from build123d import *

# Parameters (mm, degrees)
IZIM1_R                     = 3
Y_KSEKLIK_EKSTR_ZYON1_DEPTH = 3
IZIM2_R                     = 1.5
Y_KSEKLIK_EKSTR_ZYON2_DEPTH = 5
RADYUS1_R                   = 0.5
KES_EKSTR_ZYON1_DEPTH       = 2


with BuildPart() as part:
    # Çizim1 → Yükseklik-Ekstrüzyon1 (new body)
    with BuildSketch(Plane(origin=(0, 0, 0), x_dir=(1, 0, 0), z_dir=(0, 1, 0))):
        with Locations(Location((0, 0, 0), (0, 0, 270))):
            Circle(IZIM1_R)
    extrude(amount=Y_KSEKLIK_EKSTR_ZYON1_DEPTH)

    # Çizim2 → Yükseklik-Ekstrüzyon2 (add)
    with BuildSketch(Plane(origin=(0, 3, 0), x_dir=(1, 0, 0), z_dir=(0, 1, 0))):
        with Locations(Location((0, 0, 0), (0, 0, 270))):
            Circle(IZIM2_R)
    extrude(amount=Y_KSEKLIK_EKSTR_ZYON2_DEPTH)

    # Radyus1
    radyus1_edges = [part.edges().sort_by_distance(p)[0] for p in [
        (0, 0, -3),
        (0, 3, -3),
    ]]
    fillet(radyus1_edges, radius=RADYUS1_R)

    # Çizim3 → Kes-Ekstrüzyon1 (cut)
    with BuildSketch(Plane.XZ):
        Polygon((1.732050808, 0), (0.866025404, 1.5), (-0.866025404, 1.5), (-1.732050808, 0), (-0.866025404, -1.5), (0.866025404, -1.5), align=None)
    extrude(amount=-KES_EKSTR_ZYON1_DEPTH, mode=Mode.SUBTRACT)


solid = part.part
The listing builds one solid part. Answer for the finished solid, in the listing's coordinates (mm). A direction names the side the tool comes from. Round coordinates to 2 decimals unless told otherwise and drop trailing zeros. Write each loop counter-clockwise with the first axis right and the second up, starting at its lowest first coordinate (ties: lowest second). Pieces come first, ordered by that corner, then holes. Notation, with made-up numbers: M 42,48.25 L 84,48.25 A19 cw 84,84.25 Z; hole C 17.5,59 d8. An arc over 180 degrees is marked long. Write each question's results on one line, items separated by ' | '. Start each with the question number.
Item 1: For a pull along X with two mould halves and no side action, classify faces 4 (the face through (0, 2, 0)), 5 (the face through (0.9, 1.49, 2.86)), 6 (the face through (0, 0, 2)) as pulls with the +X half, pulls with the -X half, needs draft (parallel to the pull), parting line crosses it, or undercut.
Item 2: A flat-ended cylindrical pin translates along its axis: pin 1 Ø1.5 at (x, z) = (1, 0.5) entering from -Y. Find the tip coordinate at first contact, or state that the pin passes through.
Item 3: A cutting plane is placed at A-A on x = 0. Write down the section's boundary in (y, z).
Item 4: For faces 1 (the face through (0, 1, 1.5)), 2 (the face through (-2, 3, 0)), 3 (the face through (0, 8, 0)), determine the directions among +Z, -Z, +X, -X, +Y, -Y from which every point of the face is accessible in a straight line to the end or side of a thin tool.
Item 5: A cutting plane is placed at B-B on y = 6. Write down the section's boundary in (x, z).
Item 6: Straight lines are drawn through the part: L1, parallel to X at y = 1, z = -1; L2, parallel to Y at x = 2.3, z = 0; L3, parallel to Y at x = 1.25, z = -0.25. For each, find the intervals that lie inside material, in ascending order. Write a range as [from, to].
Check sheet entries:
1) face 4: undercut | face 5: parting line crosses it | face 6: needs draft
2) pin 1: y = 0
3) outline: M 0,-2.5 A0.5 ccw 0.5,-3 L 2.5,-3 A0.5 ccw 3,-2.5 L 3,-1.5 L 8,-1.5 L 8,1.5 L 3,1.5 L 3,2.5 A0.5 ccw 2.5,3 L 0.5,3 A0.5 ccw 0,2.5 L 0,1.5 L 2,1.5 L 2,-1.5 L 0,-1.5 Z
4) face 1: -Y | face 2: +Y | face 3: +Z, -Z, +X, -X, +Y
5) outline: C 0,0 d3
6) L1: [-2.83, -1.15], [1.15, 2.83] | L2: [0, 3] | L3: [2, 8]
